Autodesk Inventor part; units mm, degrees
ref_plane "YZ Plane" through (0, 0, 0) normal (1, 0, 0) x (0, 1, 0)
ref_plane "XZ Plane" through (0, 0, 0) normal (0, 1, 0) x (-1, 0, 0)
ref_plane "XY Plane" through (0, 0, 0) normal (0, 0, 1) x (1, 0, 0)
sketch "Esboço1" plane through (0, 0, 0) normal (1, 0, 0) x (0, 1, 0)
  line L0 (0, 0) -> (30, 0)
  line L1 (30, 0) -> (30, 100)
  line L2 (30, 100) -> (0, 100)
  line L3 (0, 100) -> (0, 0)
  dimension "d0" = 30
  dimension "d1" = 100
extrude "Extrusão1" add sketch "Esboço1" against normal blind 30
sketch "Esboço2" plane through (0, 0, 0) normal (1, 0, 0) x (0, 0, -1)
  point P0 (0, 0)
sketch "Esboço3" plane through (0, 30, 100) normal (0, 1, 0) x (1, 0, 0)
  line L0 (-30, 0) -> (-30, 100)
  line L1 (0, 100) -> (0, 0)
  line L2 (-30, 100) -> (0, 100)
  line L3 (0, 100) -> (0, 60)
  line L4 (0, 60) -> (-30, 60)
  line L5 (-30, 60) -> (-30, 100)
  dimension "d4" = 40
extrude "Extrusão2" add sketch "Esboço3" along normal blind 30
fillet "Arredondamento2" radius 20 2 edges at (-15, 60, 40) (-15, 60, 0)
sketch "Esboço6" plane through (0, 0, 0) normal (1, 0, 0) x (0, 0, -1)
  arc A0 (0, 40) -> (-40, 40) centre (-20, 40) ccw
  point P0 (0, 0)
hole "Furo3" at (0, 40, 20) direction (-1, 0, 0) diameter 20 end through all
properties part number "Suporte"
The listing builds one solid part. Answer for the finished solid, in the listing's coordinates (mm). A direction names the side the tool comes from. Round coordinates to 2 decimals unless told otherwise and drop trailing zeros. Loops run counter-clockwise (first coordinate to the right, second up) from the corner with the lowest first, then second, coordinate; pieces in that order, holes last.
Q1. For a pull along Z with two mould halves and no side action, classify faces 3 (the face through (-15, 35, 40)), 4 (the face through (0, 23, 51)), 5 (the face through (-15.21, 48.872, 15.386)) as released by +Z, released by -Z, zero draft, split by the parting line, or undercut.
Q2. Which of the six approach directions +Z, -Z, +X, -X, +Y, -Y give full straight-line access (tool end or side, diameter ignored) to faces 1 (the face through (-15, 15, 100)), 2 (the face through (-15, 30, 70))?
Q3. Find the intervals of material crossed by line 1 (Y direction, x = -17.5, z = 20); line 2 (Z direction, x = -7.75, y = 40); line 3 (Y direction, x = -23, z = 54), in increasing order.
Q4. Section C-C, the plane z = 26.5 is taken. Determine the outline of the cut face in (x, y).
Q5. Given pin 1 Ø1.5 at (x, z) = (-14, 14) entering from +Y; pin 2 Ø6 at (x, y) = (-13, 50.5) entering from +Z; pin 3 Ø10 at (x, z) = (-22.5, 33.5) entering from +Y, each flat-ended and moving along its own axis, determine where each tip first touches the part or whether it passes through.
Q6. Section D-D, the plane z = 75 is taken. Determine the outline of the cut face in (x, y).
Q7. Section B-B, the plane y = 47 is taken. Determine the outline of the cut face in (x, z), then the cut area to 3 significant figures.
Completed:
1. face 3: released by +Z
1. face 4: zero draft
1. face 5: undercut
2. face 1: +Z, +X, -X, +Y, -Y
2. face 2: +Z, +X, -X, +Y
3. line 1: y = 0 to 30, 50 to 60
3. line 2: z = 0 to 10, 30 to 40
3. line 3: y = 0 to 30
4. outline: (-30, 0) - (0, 0) - (0, 32.4) - (-30, 32.4) - close; (-30, 47.6) - (0, 47.6) - (0, 58.91) - (-30, 58.91) - close
5. pin 1: stops at y = 59.3
5. pin 2: stops at z = 38.54
5. pin 3: stops at y = 58.1
6. outline: (-30, 0) - (0, 0) - (0, 30) - (-30, 30) - close
7. outline: (-30, 1.26) - (0, 1.26) - (0, 12.86) - (-30, 12.86) - close; (-30, 27.14) - (0, 27.14) - (0, 38.74) - (-30, 38.74) - close
7. area: 696 mm2
